Read the model definition and answer for the solid it produces. Units are mm, in the model's axes. A direction names the side the tool comes from. Give positions to 0.01 mm unless a question says otherwise; leave off trailing zeros. Order: outer loops, then holes, each group sorted by start corner. A loop starts at its lowest first (then second) coordinate and runs counter-clockwise, first axis right, second up. Notation, with made-up numbers: M 66,42 L 86,42 A22 cw 86,59 Z; hole C 38.5,56.25 d10. An arc over 180 degrees is marked long. Write item = value, one per line. Start each with the question number.
from build123d import *

# Parameters (mm, degrees)
SKETCH028_W     = 1.3
SKETCH028_H     = 0.5
PAD004_DEPTH    = 2.9
SKETCH035_W     = 11.8
SKETCH035_H     = 4.8
POCKET013_DEPTH = 5.15
SKETCH036_W     = 1.1
SKETCH036_H     = 2.65
POCKET014_DEPTH = 0.65
SKETCH037_W     = 0.7
SKETCH037_H     = 4.8
PAD028_DEPTH    = 0.8
SKETCH038_W     = 0.85
SKETCH038_H     = 3.8
POCKET015_DEPTH = 0.65
SKETCH039_W     = 0.7
SKETCH039_H     = 0.7
POCKET016_DEPTH = 5.801


with BuildPart() as part:
    # Sketch028 → Pad004 (new body, symmetric)
    with BuildSketch(Plane.XZ):
        Polygon((6.4, 1.35), (6.4, 5.05), (-6.4, 5.05), (-6.4, 1.35), (-1.75, 1.35), (-1.75, -0.75), (1.75, -0.75), (1.75, 1.35), align=None)
        with Locations((0, 0.4)):
            Rectangle(SKETCH028_W, SKETCH028_H, mode=Mode.SUBTRACT)
    extrude(amount=PAD004_DEPTH, both=True)

    # Sketch035 (on Face6 of Pad004) → Pocket013 (cut)
    with BuildSketch(Plane(origin=(0, 0, -0.75), x_dir=(1, 0, 0), z_dir=(0, 0, -1))):
        Rectangle(SKETCH035_W, SKETCH035_H)
    extrude(amount=-POCKET013_DEPTH, mode=Mode.SUBTRACT)

    # Sketch036 (on Face3 of Pocket013) → Pocket014 (cut)
    with BuildSketch(Plane(origin=(0, 0, 5.05), x_dir=(-1, 0, 0), z_dir=(0, 0, 1))):
        with Locations((1.35, 0)):
            Rectangle(SKETCH036_W, SKETCH036_H)
    extrude(amount=-POCKET014_DEPTH, mode=Mode.SUBTRACT)

    # Sketch037 (on Face30 of Pocket014) → Pad028 (join)
    with BuildSketch(Plane(origin=(0, 0, 4.4), x_dir=(1, 0, 0), z_dir=(0, 0, -1))):
        with Locations((-2.25, 0)):
            Rectangle(SKETCH037_W, SKETCH037_H)
        with Locations((-0.45, 0)):
            Rectangle(SKETCH037_W, SKETCH037_H)
    extrude(amount=PAD028_DEPTH)

    # Sketch038 (on Face3 of Pad028) → Pocket015 (cut)
    with BuildSketch(Plane(origin=(0, 0, 5.05), x_dir=(-1, 0, 0), z_dir=(0, 0, 1))):
        with Locations((5.175, 0)):
            Rectangle(SKETCH038_W, SKETCH038_H)
    extrude(amount=-POCKET015_DEPTH, mode=Mode.SUBTRACT)

    # Sketch039 (on Face5 of Pocket015) → Pocket016 (cut, through all)
    with BuildSketch(Plane.XZ.offset(2.9)):
        with Locations((-5.15, 4.2)):
            Rectangle(SKETCH039_W, SKETCH039_H)
    extrude(amount=-POCKET016_DEPTH, mode=Mode.SUBTRACT)


solid = part.part
1) Find section A-A on z = 4.1. Determine the outline of the cut face in (x, y), plus the area to 3 significant figures.
2) Find section C-C on y = -0.25. Determine the outline of the cut face in (x, z), plus the area to 3 significant figures.
3) Find section D-D on x = -0.5. Determine the outline of the cut face in (y, z).
4) For a pull along X with two mould halves and no side action, classify faces 4 (the face through (-5.9, 0, 3)), 5 (the face through (6.4, 0, 3)), 6 (the face through (6.1, 0, 1.35)), 7 (the face through (-6.4, 0, 3)) as pulls with the +X half, pulls with the -X half, needs draft (parallel to the pull), parting line crosses it, or undercut.
5) Find section B-B on x = -5. Determine the outline of the cut face in (y, z), plus the area to 3 significant figures.
6) For faces 1 (the face through (0, 0, 5.05)), 2 (the face through (-6.2, -0.2, 1.35)), 3 (the face through (-0.8, 0, 4)), determine the directions among +Z, -Z, +X, -X, +Y, -Y from which every point of the face is accessible in a straight line to the end or side of a thin tool.
7) Find the intervals of material crossed by probe 1 along Y at (x, z) = (3.5, 1.7); probe 2 along X at (y, z) = (0.25, 3.5); probe 3 along Z at (x, y) = (1.75, 0.05), in increasing order. Write a range as [from, to].
8) Each of these flat-tipped pins is pushed along its axis until it touches: P1, Ø3, axis at x = 4.5, y = 2, coming from the -Z side; P2, Ø0.6, axis at y = 2.5, z = 0.5, coming from the -X side; P3, Ø2.5, axis at x = 3.5, y = 0, coming from the -Z side. Where does it stop, or does it pass through?
Numbers:
q1.outline = M -6.4,-2.9 L -5.5,-2.9 L -5.5,-2.4 L -5.9,-2.4 L -5.9,2.4 L -5.5,2.4 L -5.5,2.9 L -6.4,2.9 Z; M -4.8,-2.9 L 6.4,-2.9 L 6.4,2.9 L -4.8,2.9 L -4.8,2.4 L -2.6,2.4 L -2.6,-2.4 L -4.8,-2.4 Z; hole M -1.9,-2.4 L -0.8,-2.4 L -0.8,2.4 L -1.9,2.4 Z; hole M -0.1,-2.4 L 5.9,-2.4 L 5.9,2.4 L -0.1,2.4 Z
q1.area = 23.6 mm2
q2.outline = M -6.4,1.35 L -5.9,1.35 L -5.9,4.4 L -5.6,4.4 L -5.6,5.05 L -6.4,5.05 Z; M -4.75,4.4 L -2.6,4.4 L -2.6,3.6 L -1.9,3.6 L -1.9,5.05 L -4.75,5.05 Z; M -0.8,3.6 L -0.1,3.6 L -0.1,4.4 L 5.9,4.4 L 5.9,1.35 L 6.4,1.35 L 6.4,5.05 L -0.8,5.05 Z
q2.area = 11.2 mm2
q3.outline = M -2.9,-0.75 L -2.4,-0.75 L -2.4,0.15 L -2.9,0.15 Z; M -2.9,0.65 L -2.4,0.65 L -2.4,3.6 L 2.4,3.6 L 2.4,0.65 L 2.9,0.65 L 2.9,5.05 L -2.9,5.05 Z; M 2.4,-0.75 L 2.9,-0.75 L 2.9,0.15 L 2.4,0.15 Z
q4.face_4 = undercut
q4.face_5 = pulls with the +X half
q4.face_6 = needs draft
q4.face_7 = pulls with the -X half
q5.outline = M -2.9,1.35 L -2.4,1.35 L -2.4,3.85 L -2.9,3.85 Z; M -2.9,4.55 L -1.9,4.55 L -1.9,5.05 L -2.9,5.05 Z; M 1.9,4.55 L 2.9,4.55 L 2.9,5.05 L 1.9,5.05 Z; M 2.4,1.35 L 2.9,1.35 L 2.9,3.85 L 2.4,3.85 Z
q5.area = 3.50 mm2
q6.face_1 = +Z, +X, -X, +Y, -Y
q6.face_2 = -Z, -X, +Y, -Y
q6.face_3 = -Z
q7.probe_1 = [-2.9, -2.4], [2.4, 2.9]
q7.probe_2 = [-6.4, -5.9], [5.9, 6.4]
q7.probe_3 = [4.4, 5.05]
q8.P1 = 1.35
q8.P2 = -1.75
q8.P3 = 4.4
